Build history of the part. All positions in model axes, mm. A direction names the side the tool comes from. Give positions to 0.01 mm unless a question says otherwise; leave off trailing zeros. Loops run counter-clockwise (first coordinate to the right, second up) from the corner with the lowest first, then second, coordinate; pieces in that order, holes last. Notation, with made-up numbers: M 18,-39.75 L 76,-39.75 A33 ccw 76,-10.75 Z; hole C 9,7 d11. An arc over 180 degrees is marked long. Answer in a Markdown table with one row per item. Add a question column.
```python
from build123d import *

# Parameters (mm, degrees)
F0_W      = 120.686
F0_H      = 100
F0_W_2    = 76
F0_H_2    = 54
F1_DEPTH  = 10
F3_DEPTH  = 4
F4_R      = 5
F5_W      = 54.2500019073
F5_H      = 10.6249998808
F6_DEPTH  = 10
F8_DEPTH  = 1
F9_W      = 11.812498793
F9_H      = 14.8750022054
F9_W_2    = 12.2500015423
F9_W_3    = 10.9374932945
F10_DEPTH = 25
F11_R     = 5


# Not quite as in the source:
# - a feature names something its author has since deleted; it is built from what else it names


with BuildPart() as f1:
    # F0 (on Top) → F1 (new body)
    with BuildSketch(Plane.XY):
        Rectangle(F0_W, F0_H)
        Rectangle(F0_W_2, F0_H_2, mode=Mode.SUBTRACT)
    extrude(amount=F1_DEPTH)

    # F2 (on face) → F3 (join)
    with BuildSketch(Plane(origin=(0, 0, 0), x_dir=(1, 0, 0), z_dir=(0, 0, -1))):
        with BuildLine():
            ThreePointArc((55, 40), (53.5355339059, 43.5355339059), (50, 45))
            Line((50, 45), (-50, 45))
            ThreePointArc((-50, 45), (-53.5355339059, 43.5355339059), (-55, 40))
            Line((-55, 40), (-55, -40))
            ThreePointArc((-55, -40), (-53.5355339059, -43.5355339059), (-50, -45))
            Line((-50, -45), (50, -45))
            ThreePointArc((50, -45), (53.5355339059, -43.5355339059), (55, -40))
            Line((55, -40), (55, 40))
        make_face()
        with BuildLine():
            Line((-49, 44), (49, 44))
            ThreePointArc((49, 44), (52.5355339059, 42.5355339059), (54, 39))
            Line((54, 39), (54, -39))
            ThreePointArc((54, -39), (52.5355339059, -42.5355339059), (49, -44))
            Line((49, -44), (-49, -44))
            ThreePointArc((-49, -44), (-52.5355339059, -42.5355339059), (-54, -39))
            Line((-54, -39), (-54, 39))
            ThreePointArc((-54, 39), (-52.5355339059, 42.5355339059), (-49, 44))
        make_face(mode=Mode.SUBTRACT)
    extrude(amount=F3_DEPTH)

    # F4
    f4_edges = [f1.edges().sort_by_distance(p)[0] for p in [
        (-60.343, -50, 5),
        (60.343, -50, 5),
        (60.343, 50, 5),
        (-60.343, 50, 5),
        (0, 50, 10),
        (-60.343, 0, 10),
        (0, -50, 10),
        (60.343, 0, 10),
    ]]
    fillet(f4_edges, radius=F4_R)

    # F5 (on face) → F6 (join)
    with BuildSketch(Plane.XY.offset(10)):
        with Locations((0, 21.6875000596)):
            Rectangle(F5_W, F5_H)
    extrude(amount=-F6_DEPTH)

    # F7 (on face) → F8 (cut)
    with BuildSketch(Plane.XY.offset(10)):
        Polygon((48.3437515795, -40.4687528498), (48.3437515795, 36.0937528312), (27.1250009537, 36.0937528312), (27.1250009537, 27), (38, 27), (38, -27), (-38, -27), (-38, 27), (-27.1250009537, 27), (-27.1250009537, 36.0937528312), (-48.3437515795, 36.0937528312), (-48.3437515795, -40.4687528498), align=None)
    extrude(amount=-F8_DEPTH, mode=Mode.SUBTRACT)

    # F9 (on face) → F10 (cut)
    with BuildSketch(Plane.XY.offset(10)):
        with Locations((-17.0625001192, 28.6562517285)):
            Rectangle(F9_W, F9_H)
        with Locations((0, 28.6562517285)):
            Rectangle(F9_W_2, F9_H)
        with Locations((16.4062529802, 28.6562517285)):
            Rectangle(F9_W_3, F9_H)
    extrude(amount=-F10_DEPTH, mode=Mode.SUBTRACT)

    # F11
    f11_edges = [f1.edges().sort_by_distance(p)[0] for p in [
        (-27.125001, 16.375, 5),
        (27.125001, 16.375, 5),
    ]]
    fillet(f11_edges, radius=F11_R)


solid = f1.part
```
(1) Pin check, flat tips, straight feed: pin 1 (0.5 mm diameter, centred on x = -16, z = 9.5, fed in from +Y); pin 2 (2 mm diameter, centred on y = -1, z = -3, fed in from +X); pin 3 (2 mm diameter, centred on y = -8, z = -2.5, fed in from -X). Stop position of each tip, or through.
(2) Tool access for faces 4 (the cylindrical face through (-52, 43, -2)), 5 (the cylindrical face through (25.62, 17.8, 4.93)), 6 (the flat face through (-27.125, 25, 5)), 7 (the flat face through (55, 1, -2)): list every direction of +Z, -Z, +X, -X, +Y, -Y with a clear straight run to the whole face (end or side of a thin tool).
(3) Slice it at A-A, the plane x = -33.5. Give the cut face in (y, z), then the cut area to 3 significant figures.
(4) Pull direction Y, two halves, no side cores. Call faces 1 (the flat face through (-17, 21.219, 5)), 2 (the cylindrical face through (53, 44, -2)), 3 (the cylindrical face through (58.839, 0.63, 8.574)): +Y half, -Y half, draft (parallel to the pull), parting line (faces both ways), or undercut.
(5) Slice it at C-C, the plane x = 17.5. Give the cut face in (y, z) (3 decimals).
(6) Slice it at B-B, the plane y = 6.5. Give the cut face in (x, z), then the cut area to 3 significant figures.
(7) Wall check: line 1 (Y direction, x = -22.5, z = 4.5); line 2 (X direction, y = 16, z = -1.5); line 3 (X direction, y = -10.5, z = 3.75). Give the ranges that are in metal, low to high.
(8) Slice it at D-D, the plane z = 2. State how many separate pieces and enclosed holes the cut face has, then the cut area to 3 significant figures.
Solution:
| question | item | result |
|---|---|---|
| 1 | pin 1 | y = 47.63 |
| 1 | pin 2 | x = 55 |
| 1 | pin 3 | x = -55 |
| 2 | face 4 | -Z |
| 2 | face 5 | +Z, -Z |
| 2 | face 6 | +Z |
| 2 | face 7 | -Z, +X, +Y, -Y |
| 3 | outline | M -50,0 L -45,0 L -45,-4 L -44,-4 L -44,0 L -27,0 L -27,9 L -40.47,9 L -40.47,10 L -45,10 A5 ccw -50,5 Z; M 27,0 L 44,0 L 44,-4 L 45,-4 L 45,0 L 50,0 L 50,5 A5 ccw 45,10 L 36.09,10 L 36.09,9 L 27,9 Z |
| 3 | area | 435 mm^2 |
| 4 | face 1 | undercut |
| 4 | face 2 | +Y half |
| 4 | face 3 | draft |
| 5 | outline | M -50,0 L -45,0 L -45,-4 L -44,-4 L -44,0 L -27,0 L -27,9 L -40.469,9 L -40.469,10 L -45,10 A5 ccw -50,5 Z; M 16.375,0 L 21.219,0 L 21.219,10 L 16.375,10 Z; M 36.094,0 L 44,0 L 44,-4 L 45,-4 L 45,0 L 50,0 L 50,5 A5 ccw 45,10 L 36.094,10 Z |
| 6 | outline | M -60.34,0 L -55,0 L -55,-4 L -54,-4 L -54,0 L -38,0 L -38,9 L -48.34,9 L -48.34,10 L -55.34,10 A5 ccw -60.34,5 Z; M 38,0 L 54,0 L 54,-4 L 55,-4 L 55,0 L 60.34,0 L 60.34,5 A5 ccw 55.34,10 L 48.34,10 L 48.34,9 L 38,9 Z |
| 6 | area | 423 mm^2 |
| 7 | line 1 | -50 to -27, 16.39 to 21.22, 36.09 to 50 |
| 7 | line 2 | -55 to -54, 54 to 55 |
| 7 | line 3 | -60.34 to -38, 38 to 60.34 |
| 8 | separate pieces | 1 |
| 8 | enclosed holes | 4 |
| 8 | area | 7,990 mm^2 |
